Autodesk Inventor part; units mm, degrees
ref_plane "YZ Plane" through (0, 0, 0) normal (1, 0, 0) x (0, 1, 0)
ref_plane "XZ Plane" through (0, 0, 0) normal (0, 1, 0) x (-1, 0, 0)
ref_plane "XY Plane" through (0, 0, 0) normal (0, 0, 1) x (1, 0, 0)
sketch "Sketch1" plane through (0, 0, 0) normal (0, 1, 0) x (-1, 0, 0)
  line L0 (17, 21) -> (-17, 21)
  line L1 (-21, 17) -> (-21, -17)
  line L2 (-17, -21) -> (17, -21)
  line L3 (21, -17) -> (21, 17)
  line L4 (0, -30.5598) -> (0, 30.5598)
  line L5 (-30.5598, 0) -> (30.5598, 0)
  circle A0 centre (0, 0) radius 2.5
  circle A1 centre (0, 0) radius 3.5
  circle A2 centre (0, 0) radius 11
  circle A3 centre (15.5, 15.5) radius 2
  circle A4 centre (15.5, -15.5) radius 2
  circle A5 centre (-15.5, -15.5) radius 2
  circle A6 centre (-15.5, 15.5) radius 2
  arc A7 (21, 17) -> (17, 21) centre (17, 17) ccw
  arc A8 (17, -21) -> (21, -17) centre (17, -17) ccw
  arc A9 (-21, -17) -> (-17, -21) centre (-17, -17) ccw
  arc A10 (-17, 21) -> (-21, 17) centre (-17, 17) ccw
  point P0 (21, 21)
  point P1 (21, -21)
  dimension "d0" = 5
  dimension "d1" = 7
  dimension "d2" = 22
  dimension "d3" = 42
  dimension "d4" = 4
  dimension "d5" = 31
  dimension "d6" = 31
  dimension "d7" = 4
extrude "Extrusion1" add sketch "Sketch1" against normal blind 33 contours A7 L3 L5 A2 L4 L0 | L4 A2 L5 L1 A10 L0 | A2 L5 A1 L4 | L4 A1 L5 A2 | L3 A8 L2 L4 A2 L5 | A1 L5 A0 L4 | L4 A0 L5 A1 | A2 L4 A1 L5 | A2 L4 L2 A9 L1 L5 | L5 A1 L4 A2 | A1 L4 A0 L5 | L5 A0 L4 A1
extrude "Extrusion2" add sketch "Sketch1" along normal blind 2 contours A2 L5 A1 L4 | L4 A1 L5 A2 | A2 L4 A1 L5 | L5 A1 L4 A2
sketch "Sketch2" plane through (21, 0, 17) normal (1, 0, 0) x (0, 0, -1)
  line L0 (-4, 0) -> (0, 0)
  line L1 (0, -34) -> (-4, -34)
  line L2 (0, 0) -> (34, 0)
  line L3 (34, -33) -> (0, -33)
  line L4 (34, 0) -> (38, 0)
  line L5 (38, -34) -> (34, -34)
  line L6 (-4, -9) -> (2, -9)
  line L7 (2, -9) -> (2, -7)
  line L8 (2, -7) -> (32, -7)
  line L9 (32, -7) -> (32, -9)
  line L10 (32, -9) -> (38, -9)
  line L11 (-4, 0) -> (-4, -33)
  line L12 (-4, -24) -> (2, -24)
  line L13 (2, -24) -> (2, -26)
  line L14 (2, -26) -> (32, -26)
  line L15 (32, -26) -> (32, -24)
  line L16 (32, -24) -> (38, -24)
  line L17 (38, 0) -> (38, -33)
  line L18 (-4, -16.5) -> (38, -16.5) construction
  line L19 (-4, 0) -> (-4, -9)
  line L20 (-4, -24) -> (-4, -33)
  line L21 (38, 0) -> (38, -9)
  line L22 (38, -24) -> (38, -33)
  line L23 (17, -40.8) -> (17, 6.8) construction
  line L24 (-4, -9) -> (-4, -24)
  line L25 (38, -24) -> (38, -9)
  point P0 (17, 0)
  dimension "d12" = 6
  dimension "d13" = 7
  dimension "d14" = 2
extrude "Extrusion3" cut sketch "Sketch2" against normal blind 2 contours L6 L7 L8 L9 L10 L17 L16 L15 L14 L13 L12 L11
pattern_circular "Circular Pattern1" count 4 over 360 about axis through (0, 0, 0) along (0, -1, 0) of "Extrusion3"
chamfer "Chamfer1" distance 2 angle 45 4 edges at (-19, -16.5, 19) (-19, -16.5, -19) (19, -16.5, 19) (19, -16.5, -19)
sketch "Sketch3" plane through (0, -33, 0) normal (0, -1, 0) x (1, 0, 0)
  circle A0 centre (0, 0) radius 2.5
  circle A1 centre (15.5, 15.5) radius 2
  circle A2 centre (15.5, -15.5) radius 2
  circle A3 centre (-15.5, -15.5) radius 2
  circle A4 centre (-15.5, 15.5) radius 2
  line L0 (17, 21) -> (-17, 21)
  arc A5 (-17, 21) -> (-21, 17) centre (-17, 17) ccw
  line L1 (-21, 17) -> (-21, -17)
  arc A6 (-21, -17) -> (-17, -21) centre (-17, -17) ccw
  line L2 (-17, -21) -> (17, -21)
  arc A7 (17, -21) -> (21, -17) centre (17, -17) ccw
  line L3 (21, -17) -> (21, 17)
  arc A8 (21, 17) -> (17, 21) centre (17, 17) ccw
extrude "Extrusion4" add sketch "Sketch3" against normal blind 58 contours A0
chamfer "Chamfer2" distance 0.5 angle 45 4 edges at (-13.5, 0, -15.5) (-13.5, 0, 15.5) (17.5, 0, 15.5) (17.5, 0, -15.5)
fillet "Fillet1" radius 1 16 edges at (-19.8284, 0, -19.8284) (-21, 0, 0) (-19.8284, 0, 19.8284) (0, 0, 21) (19.8284, 0, 19.8284) (21, 0, 0) (19.8284, 0, -19.8284) (0, 0, -21) (19.8284, -33, 19.8284) (0, -33, 21) (-19.8284, -33, 19.8284) (-21, -33, 0) (-19.8284, -33, -19.8284) (0, -33, -21) (19.8284, -33, -19.8284) (21, -33, 0)
properties part number "NEMA 17 Stepper"
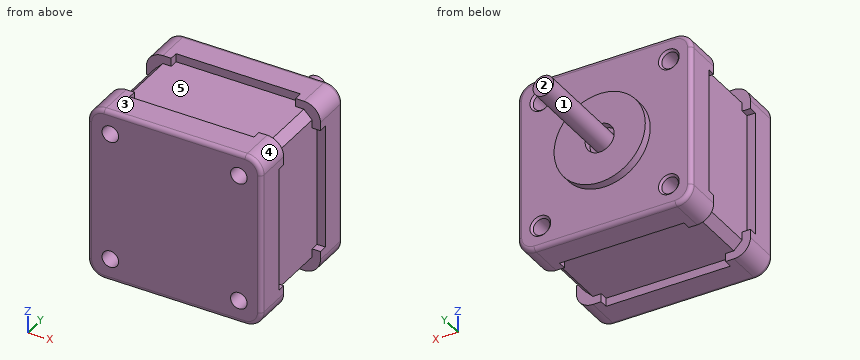
Can you work these out from the model? Positions are in its coordinate system, mm. Face numbers are marked on the shaded views. A direction names the side the tool comes from. Coordinates: 2 decimals unless noted, no trailing zeros. Loops run counter-clockwise (first coordinate to the right, second up) from the corner with the lowest first, then second, coordinate; pieces in that order, holes last.
Item 1: Suppose I cut it at B-B (z = 0). Please give me the cut outline in (x, y), then the cut area to 3 significant figures.
Answers below:
outline: (-21, -32) arc R1 ccw to (-20, -33) - (20, -33) arc R1 ccw to (21, -32) - (21, -26) - (19, -26) - (19, -7) - (21, -7) - (21, -1) arc R1 ccw to (20, 0) - (11, 0) - (11, 2) - (3.5, 2) - (3.5, 0) - (2.5, 0) - (2.5, 25) - (-2.5, 25) - (-2.5, 0) - (-3.5, 0) - (-3.5, 2) - (-11, 2) - (-11, 0) - (-20, 0) arc R1 ccw to (-21, -1) - (-21, -7) - (-19, -7) - (-19, -26) - (-21, -26) - close
area: 1,460 mm2
Item 2: I'm going to push flat-ended pins straight in: pin 1 (5 mm diameter, centred on x = 19, z = -17.5, fed in from +Y); pin 2 (1 mm diameter, centred on y = -25.5, z = 20, fed in from +X); pin 3 (3.5 mm diameter, centred on x = 15.5, z = -15.5, fed in from +Y); pin 4 (1.5 mm diameter, centred on y = -13.5, z = -4, fed in from -X). Where does each tip first touch, or does it pass through?
Answers below:
pin 1: stops at y = 0
pin 2: stops at x = 20.12
pin 3: passes through
pin 4: stops at x = -19
Item 3: Which directions (+Z, -Z, +X, -X, +Y, -Y) give clear straight access to the entire face, cutting with the end or side of a thin tool? Please do the marked faces 1 and 2.
Answers below:
face 1: +Y
face 2: +Z, -Z, +X, -X, +Y
Item 4: Please list where these lines run through material, in increasing order: L1, parallel to Z at x = 15.5, y = -10; L2, parallel to Z at x = 0, y = 0.8.
Answers below:
L1: z = -19 to -17.5, -13.5 to 13.5, 17.5 to 19
L2: z = -11 to -3.5, -2.5 to 2.5, 3.5 to 11
Item 5: Suppose I cut it at D-D (y = -2). Please give me the cut outline in (x, z), then the cut area to 3 significant figures.
Answers below:
outline: (-21, -17) arc R4 ccw to (-17, -21) - (17, -21) arc R4 ccw to (21, -17) - (21, 17) arc R4 ccw to (17, 21) - (-17, 21) arc R4 ccw to (-21, 17) - close; hole circle Ø4 at (-15.5, -15.5); hole circle Ø4 at (-15.5, 15.5); hole circle Ø4 at (15.5, -15.5); hole circle Ø4 at (15.5, 15.5)
area: 1,700 mm2
Item 6: Suppose I cut it at A-A (y = -25). Please give me the cut outline in (x, z).
Answers below:
outline: (-21, -17) arc R4 ccw to (-17, -21) - (-15, -21) - (-15, -19) - (15, -19) - (15, -21) - (17, -21) arc R4 ccw to (21, -17) - (21, -15) - (19, -15) - (19, 15) - (21, 15) - (21, 17) arc R4 ccw to (17, 21) - (15, 21) - (15, 19) - (-15, 19) - (-15, 21) - (-17, 21) arc R4 ccw to (-21, 17) - (-21, 15) - (-19, 15) - (-19, -15) - (-21, -15) - close; hole circle Ø4 at (-15.5, -15.5); hole circle Ø4 at (-15.5, 15.5); hole circle Ø4 at (15.5, -15.5); hole circle Ø4 at (15.5, 15.5)
Item 7: Suppose I cut it at C-C (x = 0). Please give me the cut outline in (y, z), then the cut area to 3 significant figures.
Answers below:
outline: (-33, -20) arc R1 ccw to (-32, -21) - (-26, -21) - (-26, -19) - (-7, -19) - (-7, -21) - (-1, -21) arc R1 ccw to (0, -20) - (0, -11) - (2, -11) - (2, -3.5) - (0, -3.5) - (0, -2.5) - (25, -2.5) - (25, 2.5) - (0, 2.5) - (0, 3.5) - (2, 3.5) - (2, 11) - (0, 11) - (0, 20) arc R1 ccw to (-1, 21) - (-7, 21) - (-7, 19) - (-26, 19) - (-26, 21) - (-32, 21) arc R1 ccw to (-33, 20) - close
area: 1,460 mm2
Item 8: If we mould it in two halves opening along X, with no side actions, what happens to the marked faces 3, 4 and 5? For each: released by +X, released by -X, zero draft, split by the parting line, or undercut.
Answers below:
face 3: zero draft
face 4: released by +X
face 5: undercut
